Design review of the part built by this model. Coordinates are the model's own, in mm. A direction names the side the tool comes from. Coordinates: 2 decimals unless noted, no trailing zeros. Write each loop counter-clockwise with the first axis right and the second up, starting at its lowest first coordinate (ties: lowest second). Pieces come first, ordered by that corner, then holes.
Q1. Add section B-B, the plane y = 15. Give the boundary of the cut face in (x, z).
Q2. To check wall thickness, follow probe 1 along X at (y, z) = (-5, -88.5); probe 2 along Y at (x, z) = (-10, -6). State the ranges of each line that lie inside material, in increasing order.
Q3. Machinability: for faces 1 (the face through (-11, 11, 0)), 2 (the face through (0, 20, -49)), which of the approach directions +Z, -Z, +X, -X, +Y, -Y give a long, thin tool a straight path to every point of the face, cutting with its end or side? Answer none if there is none.
Q4. Add section A-A, the plane x = 5. Give the boundary of the cut face in (y, z).
Q5. The part is to be moulded in two halves that separate along Y. For faces 3 (the face through (0, -20, -49)), 4 (the face through (-11, 11, -100)), 5 (the face through (0, -25, -49)), say which applies: +Y half, -Y half, draft (parallel to the pull), parting line (faces both ways), or undercut.
Q6. Add section C-C, the plane z = -44. Give the boundary of the cut face in (x, y).
from build123d import *

# Parameters (mm, degrees)
SKETCH1_W           = 50
SKETCH1_H           = 50
BOSS_EXTRUDE1_DEPTH = 100
CUT_EXTRUDE1_DEPTH  = 400


with BuildPart() as part:
    # Sketch1 → Boss-Extrude1 (new body)
    with BuildSketch(Plane.XY):
        Rectangle(SKETCH1_W, SKETCH1_H)
    extrude(amount=-BOSS_EXTRUDE1_DEPTH)

    # Sketch2 → Cut-Extrude1 (cut)
    with BuildSketch(Plane.XY):
        Polygon((7.5, 7.5), (20, 7.5), (20, -7.5), (7.5, -7.5), (7.5, -20), (-7.5, -20), (-7.5, -7.5), (-20, -7.5), (-20, 7.5), (-7.5, 7.5), (-7.5, 20), (7.5, 20), align=None)
    extrude(amount=-CUT_EXTRUDE1_DEPTH, mode=Mode.SUBTRACT)


solid = part.part
Here are the results:
1. outline: (-25, -100) - (-7.5, -100) - (-7.5, 0) - (-25, 0) - close; (7.5, -100) - (25, -100) - (25, 0) - (7.5, 0) - close
2. probe 1: x = -25 to -20, 20 to 25
2. probe 2: y = -25 to -7.5, 7.5 to 25
3. face 1: +Z, +X, -X, +Y, -Y
3. face 2: +Z, -Z
4. outline: (-25, -100) - (-20, -100) - (-20, 0) - (-25, 0) - close; (20, -100) - (25, -100) - (25, 0) - (20, 0) - close
5. face 3: undercut
5. face 4: draft
5. face 5: -Y half
6. outline: (-25, -25) - (25, -25) - (25, 25) - (-25, 25) - close; hole (-20, -7.5) - (-7.5, -7.5) - (-7.5, -20) - (7.5, -20) - (7.5, -7.5) - (20, -7.5) - (20, 7.5) - (7.5, 7.5) - (7.5, 20) - (-7.5, 20) - (-7.5, 7.5) - (-20, 7.5) - close
